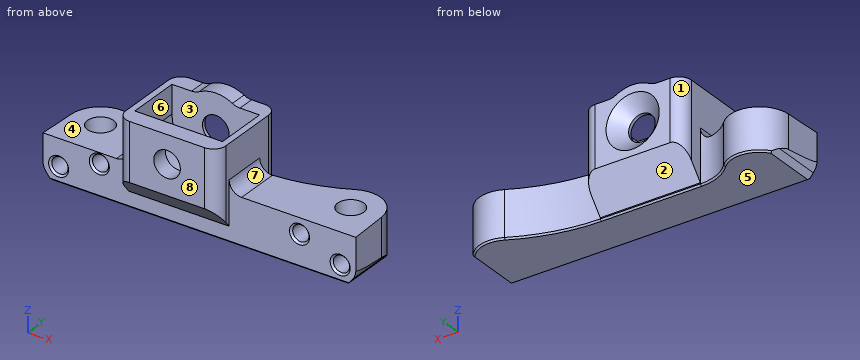
```python
from build123d import *

# Parameters (mm, degrees)
BOSS_EXTRUDE1_DEPTH                             = 16
SKETCH2_R                                       = 4.25
CUT_EXTRUDE1_DEPTH                              = 28.6
CUT_EXTRUDE2_START                              = -5.3
CUT_EXTRUDE2_DEPTH                              = 17
CSK_FOR_M8_FLAT_HEAD_MACHINE_SCREW1_D           = 8
CSK_FOR_M8_FLAT_HEAD_MACHINE_SCREW1_CSINK_D     = 17
CSK_FOR_M8_FLAT_HEAD_MACHINE_SCREW1_CSINK_ANGLE = 90
SKETCH6_R                                       = 4.2
BOSS_EXTRUDE2_DEPTH                             = 15
SKETCH7_R                                       = 4.2
BOSS_EXTRUDE3_DEPTH                             = 4
SKETCH9_R                                       = 2.6
CUT_EXTRUDE3_DEPTH                              = 6
CUT_EXTRUDE4_DEPTH                              = 1.5
FILLET2_R                                       = 4
FILLET3_R                                       = 4
BOSS_EXTRUDE4_DEPTH                             = 5.3
FILLET4_R                                       = 5
CHAMFER1_SIZE                                   = 0.6
CUT_EXTRUDE5_DEPTH                              = 23.1
CHAMFER2_SIZE                                   = 0.5


with BuildPart() as part:
    # Sketch1 → Boss-Extrude1 (new body, symmetric)
    with BuildSketch(Plane(origin=(0, 0, 0), x_dir=(0, 0, -1), z_dir=(1, 0, 0))):
        Polygon((0, 0), (0, 14), (-0.8467959, 14), (-10.5, 22.1), (-30, 22.1), (-30, -5.5), (-11.5, -5.5), (-4.945355241, 0), align=None)
    extrude(amount=BOSS_EXTRUDE1_DEPTH, both=True)

    # Sketch2 → Cut-Extrude1 (cut, through all)
    with BuildSketch(Plane(origin=(0, 22.1, 0), x_dir=(1, 0, 0), z_dir=(0, 1, 0))):
        with Locations(Location((0, -21, 0), (0, 0, 270))):  # turned: the seam where the file's is
            Circle(SKETCH2_R)
    extrude(amount=-CUT_EXTRUDE1_DEPTH, mode=Mode.SUBTRACT)

    # Sketch3 → Cut-Extrude2 (cut)
    with BuildSketch(Plane(origin=(0, 22.1, 0), x_dir=(1, 0, 0), z_dir=(0, 1, 0)).offset(CUT_EXTRUDE2_START)):
        with BuildLine():
            Line((-14, -21), (-14, -59.082734499))
            Line((-14, -59.082734499), (14, -59.082734499))
            Line((14, -59.082734499), (14, -21))
            ThreePointArc((14, -21), (0, -7), (-14, -21))
        make_face()
    extrude(amount=-CUT_EXTRUDE2_DEPTH, mode=Mode.SUBTRACT)

    # CSK for M8 Flat Head Machine Screw1 (through all)
    with Locations(Plane(origin=(0, 22.1, 0), x_dir=(-1, 0, 0), z_dir=(0, 1, 0))):
        with Locations((0, 21)):
            CounterSinkHole(CSK_FOR_M8_FLAT_HEAD_MACHINE_SCREW1_D / 2, CSK_FOR_M8_FLAT_HEAD_MACHINE_SCREW1_CSINK_D / 2, counter_sink_angle=CSK_FOR_M8_FLAT_HEAD_MACHINE_SCREW1_CSINK_ANGLE)

    # Sketch6 → Boss-Extrude2 (add)
    with BuildSketch(Plane(origin=(0, 0, 0), x_dir=(-1, 0, 0), z_dir=(0, 0, -1))):
        with BuildLine():
            Line((-16, 14), (-16, 0))
            Line((-16, 0), (-56.5, 0))
            Line((-56.5, 0), (-55.992024719, 12.389187266))
            ThreePointArc((-55.992024719, 12.389187266), (-51.251583122, 20.226327117), (-42.094272681, 20.41662443))
            ThreePointArc((-42.094272681, 20.41662443), (-29.435811623, 15.627699401), (-16, 14))
        make_face()
        with Locations((-46.5, 12)):
            Circle(SKETCH6_R, mode=Mode.SUBTRACT)
        with BuildLine():
            Line((42.992024719, 12.389187266), (43.5, 0))
            Line((43.5, 0), (16, 0))
            Line((16, 0), (16, 14))
            ThreePointArc((16, 14), (21.777483046, 15.185872893), (26.620689655, 18.551724138))
            ThreePointArc((26.620689655, 18.551724138), (36.846757278, 20.890962587), (42.992024719, 12.389187266))
        make_face()
        with Locations((33.5, 12)):
            Circle(SKETCH6_R, mode=Mode.SUBTRACT)
    extrude(amount=-BOSS_EXTRUDE2_DEPTH)

    # Sketch7 → Boss-Extrude3 (add)
    with BuildSketch(Plane(origin=(0, 0, 0), x_dir=(-1, 0, 0), z_dir=(0, 0, -1))):
        with Locations((-46.5, 12)):
            Circle(SKETCH7_R)
        with Locations((33.5, 12)):
            Circle(SKETCH7_R)
    extrude(amount=-BOSS_EXTRUDE3_DEPTH)

    # Sketch9 → Cut-Extrude3 (cut)
    with BuildSketch(Plane.XZ):
        with Locations(Location((-38.5, 5, 0), (0, 0, 270))):  # turned: the seam where the file's is
            Circle(SKETCH9_R)
        with Locations(Location((-25.5, 10, 0), (0, 0, 270))):  # turned: the seam where the file's is
            Circle(SKETCH9_R)
        with Locations(Location((38.5, 10, 0), (0, 0, 270))):  # turned: the seam where the file's is
            Circle(SKETCH9_R)
        with Locations(Location((51.5, 5, 0), (0, 0, 270))):  # turned: the seam where the file's is
            Circle(SKETCH9_R)
    extrude(amount=-CUT_EXTRUDE3_DEPTH, mode=Mode.SUBTRACT)

    # Sketch11 → Cut-Extrude4 (cut)
    with BuildSketch(Plane.XY.offset(15)):
        with BuildLine():
            Line((-42.992024719, 12.389187266), (-43.5, 0))
            Line((-43.5, 0), (-16, 0))
            Line((-16, 0), (-16, 14))
            ThreePointArc((-16, 14), (-21.777483046, 15.185872893), (-26.620689655, 18.551724138))
            ThreePointArc((-26.620689655, 18.551724138), (-36.846757278, 20.890962587), (-42.992024719, 12.389187266))
        make_face()
    extrude(amount=-CUT_EXTRUDE4_DEPTH, mode=Mode.SUBTRACT)

    # Fillet2
    fillet2_edges = [part.edges().sort_by_distance(p)[0] for p in [
        (-16, 7, 13.5),
        (16, 7, 15),
    ]]
    fillet(fillet2_edges, radius=FILLET2_R)

    # Fillet3
    fillet3_edges = [part.edges().sort_by_distance(p)[0] for p in [
        (16, -5.5, 20.75),
        (-16, -5.5, 20.75),
        (-16, 22.1, 20.25),
        (16, 22.1, 20.25),
    ]]
    fillet(fillet3_edges, radius=FILLET3_R)

    # Sketch10 → Boss-Extrude4 (add)
    with BuildSketch(Plane(origin=(0, 22.1, 0), x_dir=(1, 0, 0), z_dir=(0, 1, 0))):
        with BuildLine():
            Line((6.32455532, -30), (-6.32455532, -30))
            ThreePointArc((-6.32455532, -30), (0, -32), (6.32455532, -30))
        make_face()
    extrude(amount=-BOSS_EXTRUDE4_DEPTH)

    # Fillet4
    fillet4_edges = [part.edges().sort_by_distance(p)[0] for p in [
        (6.32455532, 19.45, 30),
        (-6.32455532, 19.45, 30),
    ]]
    fillet(fillet4_edges, radius=FILLET4_R)

    # Chamfer1
    chamfer1_edges = [part.edges().sort_by_distance(p)[0] for p in [
        (-38.5, 0, 7.6),
        (-25.5, 0, 12.6),
        (38.5, 0, 12.6),
        (51.5, 0, 7.6),
    ]]
    chamfer(chamfer1_edges, length=CHAMFER1_SIZE)

    # Sketch12 → Cut-Extrude5 (cut, through all)
    with BuildSketch(Plane.XZ):
        with BuildLine():
            Line((-42.330222216, 1.786061952), (-40.831538291, 0))
            Line((-40.831538291, 0), (-43.5, 0))
            Line((-43.5, 0), (-43.5, 5))
            ThreePointArc((-43.5, 5), (-43.198463104, 3.289899283), (-42.330222216, 1.786061952))
        make_face()
        with BuildLine():
            Line((55.330222216, 1.786061952), (53.831538291, 0))
            Line((53.831538291, 0), (56.5, 0))
            Line((56.5, 0), (56.5, 5))
            ThreePointArc((56.5, 5), (56.198463104, 3.289899283), (55.330222216, 1.786061952))
        make_face()
    extrude(amount=-CUT_EXTRUDE5_DEPTH, mode=Mode.SUBTRACT)

    # Chamfer2
    chamfer2_edges = [part.edges().sort_by_distance(p)[0] for p in [
        (-33.840931852, 21.493880422, 0),
        (-21.777483046, 15.185872893, 0),
        (0, 14, 0),
        (29.435811623, 15.627699401, 0),
        (48.384280249, 21.311255981, 0),
        (6.5, 0, 0),
    ]]
    chamfer(chamfer2_edges, length=CHAMFER2_SIZE)


solid = part.part
```
Part model, mm, in its own coordinate system. Face numbers are marked on the shaded views. A direction names the side the tool comes from. Round coordinates to 2 decimals unless told otherwise and drop trailing zeros. Loops run counter-clockwise (first coordinate to the right, second up) from the corner with the lowest first, then second, coordinate; pieces in that order, holes last.
1. Drill centre lines: line 1 along Y through (x, z) = (46.5, 11.75); line 2 along X through (y, z) = (2.8, 10); line 3 along X through (y, z) = (0.5, 26). Where is each one in solid material? Low to high.
Solutions:
line 1: y = 0 to 7.8, 16.2 to 21.5
line 2: x = -43.39 to -28.1, -22.9 to -8.66, 8.66 to 35.9, 41.1 to 56.39
line 3: x = -16 to -14, 14 to 16
2. Slice it at B-B (y = 8.75). Give the cut face in (x, z), and give its area (3 significant figures).
Solutions:
outline: (-43.14, 3.14) arc R5 ccw to (-42.33, 1.79) - (-40.83, 0) - (53.83, 0) - (55.33, 1.79) arc R5 ccw to (56.14, 3.14) - (56.14, 15) - (49.16, 15) - (49.16, 4) - (43.84, 4) - (43.84, 15) - (20, 15) arc R4 cw to (16, 19) - (16, 30) - (14, 30) - (14, 21) arc R14 cw to (-14, 21) - (-14, 30) - (-16, 30) - (-16, 17.5) arc R4 cw to (-20, 13.5) - (-30.84, 13.5) - (-30.84, 4) - (-36.16, 4) - (-36.16, 13.5) - (-43.14, 13.5) - close
area: 1,260 mm2
3. Two-plate mould, pull along Y, no slides. Class the marked faces 6, 7 and 8: pulls with the +Y half, pulls with the -Y half, needs draft (parallel to the pull), parting line crosses it, or undercut.
Solutions:
face 6: undercut
face 7: needs draft
face 8: pulls with the -Y half
4. Flat gauge pins, fed straight in: pin 1 (7 mm diameter, centred on x = -25.5, z = 10, fed in from -Y); pin 2 (6.5 mm diameter, centred on x = 44, y = 16, fed in from +Z); pin 3 (4 mm diameter, centred on y = 2.5, z = 19, fed in from -X); pin 4 (7 mm diameter, centred on x = 0, z = 21, fed in from -Y). Where does each tip first touch, or does it go through?
Solutions:
pin 1: stops at y = 0
pin 2: stops at z = 15
pin 3: stops at x = -16.03
pin 4: passes through
5. Slice it at A-A (x = 46.5). Give the cut face in (y, z).
Solutions:
outline: (0, 0.5) - (0.5, 0) - (21, 0) - (21.5, 0.5) - (21.5, 15) - (16.2, 15) - (16.2, 4) - (7.8, 4) - (7.8, 15) - (0, 15) - close
6. 3-axis set-ups, long thin cutter, end or side, ignore diameter. For the marked faces 1, 2, 3, 4 and 5: which of +Z, -Z, +X, -X, +Y, -Y reach the whole face in a straight line?
Solutions:
face 1: +Z, -Z, +Y
face 2: -Z, +Y
face 3: +Z
face 4: +Z, -X, +Y, -Y
face 5: -Z, +X, -X, +Y, -Y
